Geometry: final body of the model. Coordinates: model frame, mm. Coordinates: 2 decimals unless noted, no trailing zeros. Write each loop counter-clockwise with the first axis right and the second up, starting at its lowest first coordinate (ties: lowest second). Pieces come first, ordered by that corner, then holes. Notation, with made-up numbers: (-8.5, -26) -> (48.5, -26) arc R17 cw to (48.5, 5) -> close; hole circle Ø4 at (50.25, 13.25). An arc over 180 degrees is marked (long way). One line per item, written item: value.
```python
from build123d import *

# Parameters (mm, degrees)
CYLINDER006_R     = 14
CYLINDER006_DEPTH = 1
CYLINDER005_R     = 0.4
CYLINDER005_DEPTH = 1
CYLINDER001_R     = 12.6
CYLINDER001_DEPTH = 8
CYLINDER_R        = 15
CYLINDER_DEPTH    = 8
CYLINDER002_R     = 15
CYLINDER002_DEPTH = 1
FILLET_R          = 0.7
FILLET001_R       = 0.7
FILLET002_R       = 0.8
CYLINDER004_R     = 0.4
CYLINDER004_DEPTH = 0.6
CYLINDER003_R     = 0.65
CYLINDER003_DEPTH = 0.6
CHAMFER_SIZE      = 0.2
CYLINDER007_R     = 14
CYLINDER007_DEPTH = 1


with BuildPart() as cylinder006:
    # Cylinder006 → Cylinder006 (new body)
    with BuildSketch(Plane.XY.offset(7)):
        Circle(CYLINDER006_R)
    extrude(amount=CYLINDER006_DEPTH)


with BuildPart() as cylinder005:
    # Cylinder005 → Cylinder005 (new body)
    with BuildSketch(Plane.XY):
        Circle(CYLINDER005_R)
    extrude(amount=CYLINDER005_DEPTH)


with BuildPart() as cylinder001:
    # Cylinder001 → Cylinder001 (new body)
    with BuildSketch(Plane.XY):
        Circle(CYLINDER001_R)
    extrude(amount=CYLINDER001_DEPTH)


with BuildPart() as cut:
    # Cylinder → Cylinder (new body)
    with BuildSketch(Plane.XY):
        Circle(CYLINDER_R)
    extrude(amount=CYLINDER_DEPTH)

    # Cut: cut Cylinder001
    add(cylinder001.part, mode=Mode.SUBTRACT)


with BuildPart() as fillet002:
    # Cylinder002 → Cylinder002 (new body)
    with BuildSketch(Plane.XY):
        Circle(CYLINDER002_R)
    extrude(amount=CYLINDER002_DEPTH)

    # Fusion: union Cut
    add(cut.part)

    # Cut001: cut Cylinder005
    add(cylinder005.part, mode=Mode.SUBTRACT)

    # Cut003: cut Cylinder006
    add(cylinder006.part, mode=Mode.SUBTRACT)

    # Fillet
    fillet_edges = [fillet002.edges().sort_by_distance(p)[0] for p in [
        (-15, 0, 8),
    ]]
    fillet(fillet_edges, radius=FILLET_R)

    # Fillet001
    fillet001_edges = [fillet002.edges().sort_by_distance(p)[0] for p in [
        (-15, 0, 0),
    ]]
    fillet(fillet001_edges, radius=FILLET001_R)

    # Fillet002
    fillet002_edges = [fillet002.edges().sort_by_distance(p)[0] for p in [
        (-0.4, 0, 0),
    ]]
    fillet(fillet002_edges, radius=FILLET002_R)


with BuildPart() as cylinder004:
    # Cylinder004 → Cylinder004 (new body)
    with BuildSketch(Plane.XY.offset(1)):
        Circle(CYLINDER004_R)
    extrude(amount=CYLINDER004_DEPTH)


with BuildPart() as chamfer_body:
    # Cylinder003 → Cylinder003 (new body)
    with BuildSketch(Plane.XY.offset(1)):
        Circle(CYLINDER003_R)
    extrude(amount=CYLINDER003_DEPTH)

    # Cut002: cut Cylinder004
    add(cylinder004.part, mode=Mode.SUBTRACT)

    # Chamfer
    chamfer_edges = [chamfer_body.edges().sort_by_distance(p)[0] for p in [
        (-0.65, 0, 1.6),
    ]]
    chamfer(chamfer_edges, length=CHAMFER_SIZE)


with BuildPart() as cone:
    # Cone → Cone (revolve)
    with BuildSketch(Plane(origin=(0, 0, 7), x_dir=(1, 0, 0), z_dir=(0, -1, 0))):
        Polygon((0, 0), (13.8, 0), (14, 1), (0, 1), align=None)
    revolve(axis=Axis((0, 0, 7), (0, 0, 1)))


with BuildPart() as fusion001:
    # Cylinder007 → Cylinder007 (new body)
    with BuildSketch(Plane.XY.offset(7)):
        Circle(CYLINDER007_R)
    extrude(amount=CYLINDER007_DEPTH)

    # Cut004: cut Cone
    add(cone.part, mode=Mode.SUBTRACT)

    # Fusion001: union Fillet002, Chamfer body
    add(fillet002.part)
    add(chamfer_body.part)


with BuildPart() as fusion001_1:
    # Fusion001 placement: moved
    add(fusion001.part.moved(Location((0, 0, 3.35))))


solid = fusion001_1.part
```
(1) First-contact query: pin 1 (1 mm diameter, centred on x = 0, y = 0, fed in from +Z); pin 2 (3 mm diameter, centred on x = 12, z = 9.5, fed in from -Y); pin 3 (1 mm diameter, centred on x = 3.5, z = 6.5, fed in from -Y). Flat tips, straight axial feed; report the tip coordinate or a pass-through.
Responses:
pin 1: stops at z = 4.95
pin 2: stops at y = -10.71
pin 3: stops at y = -14.7
(2) Section C-C (z = 9.75). Return the cut outline in (x, y), then the cut area to 3 significant figures.
Responses:
outline: circle Ø30 at (0, 0); hole circle Ø25.2 at (0, 0)
area: 208 mm2
(3) Pull-direction query (Y, two-part tool) for faces 1 (the flat face through (6.1, -11.2, 10.35)), 2 (the cylindrical face through (-0.085, 0.644, 4.547)), 3 (the cylindrical face through (-14.985, 0.66, 7.304)), 4 (the flat face through (3, 0, 3.35)); classes: released by +Y, released by -Y, zero draft, split by the parting line, or undercut.
Responses:
face 1: undercut
face 2: undercut
face 3: split by the parting line
face 4: zero draft
(4) Line query: line 1 (Y direction, x = 0, z = 4.55); line 2 (Y direction, x = 0, z = 4.3); line 3 (Z direction, x = -6.5, y = 11.5). Output: solid intervals per line, ascending. Write a range as [from, to].
Responses:
line 1: y = [-15, -12.6], [-0.65, -0.4], [0.4, 0.65], [12.6, 15]
line 2: y = [-15, -0.4], [0.4, 15]
line 3: z = [3.35, 10.35]
(5) Section A-A (x = 0). Return the cut outline in (y, z), then the cut area to 3 significant figures.
Responses:
outline: (-15, 4.05) arc R0.7 ccw to (-14.3, 3.35) -> (-1.2, 3.35) arc R0.8 ccw to (-0.4, 4.15) -> (-0.4, 4.95) -> (-0.45, 4.95) -> (-0.65, 4.75) -> (-0.65, 4.35) -> (-12.6, 4.35) -> (-12.6, 10.35) -> (-13.8, 10.35) -> (-14, 11.35) -> (-14.3, 11.35) arc R0.7 ccw to (-15, 10.65) -> close; (0.4, 4.15) arc R0.8 ccw to (1.2, 3.35) -> (14.3, 3.35) arc R0.7 ccw to (15, 4.05) -> (15, 10.65) arc R0.7 ccw to (14.3, 11.35) -> (14, 11.35) -> (13.8, 10.35) -> (12.6, 10.35) -> (12.6, 4.35) -> (0.65, 4.35) -> (0.65, 4.75) -> (0.45, 4.95) -> (0.4, 4.95) -> close
area: 59.8 mm2
